Input: dimensioned drawing with shaded views. Units: mm. Origin: part minimum x, y, z. Round coordinates to 2 decimals unless told otherwise and drop trailing zeros. Loops run counter-clockwise (first coordinate to the right, second up) from the corner with the lowest first, then second, coordinate; pieces in that order, holes last.
Item 1: Section query A-A on y = 7. Return loops of the section in (x, z).
Item 2: Ray query, L1, parallel to X at y = 9, z = 8 (1 decimal); L2, parallel to X at y = 10.5, z = 63.5; L3, parallel to Z at x = 107.5, y = 10 (1 decimal). Return the intervals inside material, ascending.
Item 3: Section query B-B on z = 5.5. Return loops of the section in (x, y), then the cut area to 3 significant figures.
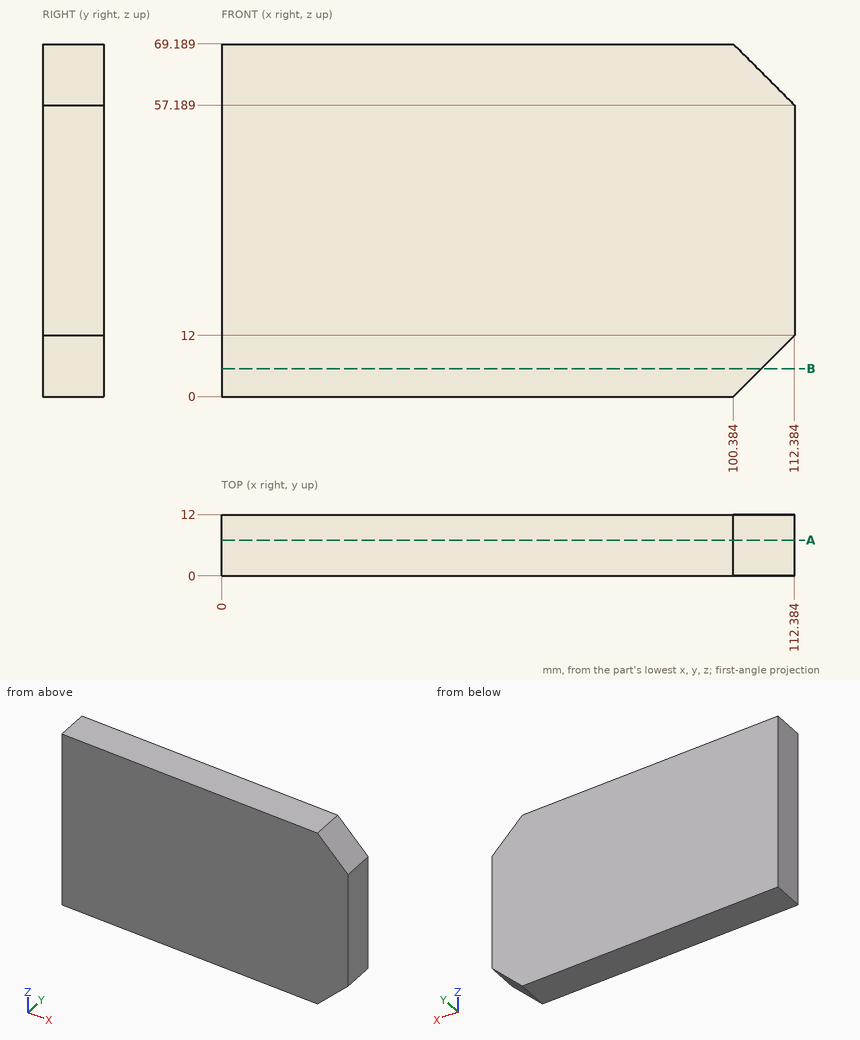
Data:
1. outline: (0, 0) - (100.38, 0) - (112.38, 12) - (112.38, 57.19) - (100.38, 69.19) - (0, 69.19) - close
2. L1: x = 0 to 108.4
2. L2: x = 0 to 106.07
2. L3: z = 7.1 to 62.1
3. outline: (0, 0) - (105.88, 0) - (105.88, 12) - (0, 12) - close
3. area: 1,270 mm2
